Autodesk Inventor part; units mm, degrees
ref_plane "YZ Plane" through (0, 0, 0) normal (1, 0, 0) x (0, 1, 0)
ref_plane "XZ Plane" through (0, 0, 0) normal (0, 1, 0) x (-1, 0, 0)
ref_plane "XY Plane" through (0, 0, 0) normal (0, 0, 1) x (1, 0, 0)
sketch "Sketch1" plane through (0, 0, 0) normal (0, 0, 1) x (1, 0, 0)
  line L0 (-40, 5) -> (0, 5)
  line L1 (0, 5) -> (0, -5)
  line L2 (0, -5) -> (-40, -5)
  line L3 (-40, -5) -> (-40, 5)
  line L4 (-10, 35) -> (0, 35)
  line L5 (0, 35) -> (0, 5)
  line L6 (0, 5) -> (-10, 5)
  line L7 (-10, 5) -> (-10, 35)
  point P0 (0, 0)
  point P1 (0, 5)
  dimension "d0" = 10
  dimension "d1" = 40
  dimension "d2" = 40
extrude "Extrusion1" add sketch "Sketch1" along normal blind 40
sketch "Sketch2" plane through (-10, 5, 0) normal (-1, 0, 0) x (0, 0, 1)
  line L0 (8.5, 20) -> (11.5, 20) construction
  line L1 (8.5, 17) -> (11.5, 17)
  line L2 (11.5, 23) -> (8.5, 23)
  arc A0 (8.5, 23) -> (8.5, 17) centre (8.5, 20) ccw
  arc A1 (11.5, 17) -> (11.5, 23) centre (11.5, 20) ccw
  line L3 (0, 30) -> (0, 0)
  line L4 (0, 30) -> (40, 30)
  line L5 (20, 21.547) -> (20, 15) construction
  line L6 (31.5, 20) -> (28.5, 20) construction
  line L7 (31.5, 17) -> (28.5, 17)
  line L8 (28.5, 23) -> (31.5, 23)
  arc A2 (31.5, 17) -> (31.5, 23) centre (31.5, 20) ccw
  arc A3 (28.5, 23) -> (28.5, 17) centre (28.5, 20) ccw
  point P0 (0, -5)
  point P1 (10, 20)
  point P2 (20, 18.2735)
  point P3 (20, 30)
  point P4 (30, 20)
  dimension "d5" = 6
  dimension "d6" = 3
  dimension "d7" = 10
  dimension "d8" = 10
extrude "Extrusion2" cut sketch "Sketch2" against normal through all
sketch "Sketch3" plane through (-40, 5, 0) normal (0, 1, 0) x (1, 0, 0)
  line L0 (10, -8.5) -> (10, -11.5) construction
  line L1 (7, -8.5) -> (7, -11.5)
  line L2 (13, -11.5) -> (13, -8.5)
  arc A0 (13, -8.5) -> (7, -8.5) centre (10, -8.5) ccw
  arc A1 (7, -11.5) -> (13, -11.5) centre (10, -11.5) ccw
  line L3 (30, 0) -> (0, 0)
  line L4 (0, 0) -> (0, -40)
  line L5 (15.2557, -20) -> (9.287, -20) construction
  line L6 (10, -31.5) -> (10, -28.5) construction
  line L7 (7, -31.5) -> (7, -28.5)
  line L8 (13, -28.5) -> (13, -31.5)
  arc A2 (7, -31.5) -> (13, -31.5) centre (10, -31.5) ccw
  arc A3 (13, -28.5) -> (7, -28.5) centre (10, -28.5) ccw
  point P0 (40, 0)
  point P1 (10, -10)
  point P2 (12.2713, -20)
  point P3 (0, -20)
  point P4 (10, -30)
  dimension "d11" = 3
  dimension "d12" = 6
  dimension "d13" = 10
  dimension "d14" = 10
extrude "Extrusion3" cut sketch "Sketch3" against normal through all
chamfer "Chamfer1" distance 10 angle 45 1 edges at (-10, 5, 20)
fillet "Fillet1" radius 2 5 edges at (-10, 35, 20) (0, 35, 20) (0, -5, 20) (-40, -5, 20) (-40, 5, 20)
equation "\"d2\" = d1"
properties part number "0008-10-022 Suport L" material "ABS Plastic"
Here's how the part is built. I have some questions about the finished solid (model axes, mm). A direction names the side the tool comes from. Coordinates: 2 decimals unless noted, no trailing zeros. Write each loop counter-clockwise with the first axis right and the second up, starting at its lowest first coordinate (ties: lowest second). Pieces come first, ordered by that corner, then holes.
1) Which directions (+Z, -Z, +X, -X, +Y, -Y) give clear straight access to the entire face, cutting with the end or side of a thin tool? Please do faces 4 (the face through (-27, 0, 10)), 5 (the face through (-5.1, 25.1, 25.5)), 6 (the face through (-11, 6, 0)).
Filled in:
face 4: +Y, -Y
face 5: +X, -X
face 6: -Z, +X, -X, +Y, -Y
2) If we section it at D-D (y = 2): List the corners of the cut face in (x, z) for me.
Filled in:
outline: (-40, 0) - (0, 0) - (0, 40) - (-40, 40) - close; hole (-33, 8.5) arc R3 ccw to (-27, 8.5) - (-27, 11.5) arc R3 ccw to (-33, 11.5) - close; hole (-33, 28.5) arc R3 ccw to (-27, 28.5) - (-27, 31.5) arc R3 ccw to (-33, 31.5) - close
3) If we section it at B-B (y = 25): List the corners of the cut face in (x, z) for me, plus the area to 3 significant figures.
Filled in:
outline: (-10, 0) - (0, 0) - (0, 5.5) - (-10, 5.5) - close; (-10, 14.5) - (0, 14.5) - (0, 25.5) - (-10, 25.5) - close; (-10, 34.5) - (0, 34.5) - (0, 40) - (-10, 40) - close
area: 220 mm2
4) If I drill on line 1 (Y direction, x = -36, z = 19); line 2 (X direction, y = 30.5, z = 22); line 3 (X direction, y = 6, z = 22), over which ranges is the centre line in solid material (lowest first)?
Filled in:
line 1: y = -5 to 5
line 2: x = -10 to 0
line 3: x = -19 to 0
5) I'm going to push flat-ended pins straight in: pin 1 (4 mm diameter, centred on y = 22.5, z = 7, fed in from -X); pin 2 (1 mm diameter, centred on y = 4, z = 23, fed in from -X); pin 3 (8 mm diameter, centred on x = -24.5, z = 5, fed in from +Y); pin 4 (2 mm diameter, centred on x = -28.5, y = 7.5, fed in from +Z). Where does each tip first touch, or does it pass through?
Filled in:
pin 1: stops at x = -10
pin 2: stops at x = -39.94
pin 3: stops at y = 5
pin 4: passes through
6) If we section it at A-A (x = -30): List the corners of the cut face in (y, z) for me, plus the area to 3 significant figures.
Filled in:
outline: (-5, 0) - (5, 0) - (5, 5.5) - (-5, 5.5) - close; (-5, 14.5) - (5, 14.5) - (5, 25.5) - (-5, 25.5) - close; (-5, 34.5) - (5, 34.5) - (5, 40) - (-5, 40) - close
area: 220 mm2
7) Thinking about a two-plate mould opening in Y: for faces 1 (the face through (-30.1, 0.1, 34.5)), 2 (the face through (-5, 28, 30)), 3 (the face through (-9.4, 34.43, 20.28)), which applies, +Y half, -Y half, draft (parallel to the pull), parting line (faces both ways), or undercut?
Filled in:
face 1: draft
face 2: undercut
face 3: +Y half
8) If we section it at C-C (z = 32.5): List the corners of the cut face in (x, y) for me, plus the area to 3 significant figures.
Filled in:
outline: (-40, -3) arc R2 ccw to (-38, -5) - (-32.83, -5) - (-32.83, 5) - (-38, 5) arc R2 ccw to (-40, 3) - close; (-27.17, -5) - (-2, -5) arc R2 ccw to (0, -3) - (0, 22.17) - (-10, 22.17) - (-10, 15) - (-20, 5) - (-27.17, 5) - close; (-10, 27.83) - (0, 27.83) - (0, 33) arc R2 ccw to (-2, 35) - (-8, 35) arc R2 ccw to (-10, 33) - close
area: 633 mm2
